from build123d import *

# Parameters (mm, degrees)
F0_W      = 76.2
F0_H      = 101.6
F1_DEPTH  = 25.4
F2_W      = 76.2
F2_H      = 101.6
F2_R      = 6.35
F3_DEPTH  = 25.4
F4_W      = 25.4
F4_H      = 50.8
F6_W      = 18.3004425924
F6_H      = 12.7
F8_R      = 2.54
F9_SIZE   = 2.54
F10_DEPTH = 25.4


with BuildPart() as f1:
    # F0 (on Top) → F1 (new body)
    with BuildSketch(Plane.XY):
        Rectangle(F0_W, F0_H)
    extrude(amount=F1_DEPTH)

    # F2 (on face) → F3 (join)
    with BuildSketch(Plane.XY.offset(25.4)):
        Rectangle(F2_W, F2_H)
        with Locations((-25.4, -38.1)):
            Circle(F2_R, mode=Mode.SUBTRACT)
        with Locations((25.4, -38.1)):
            Circle(F2_R, mode=Mode.SUBTRACT)
        with Locations((-25.4, 38.1)):
            Circle(F2_R, mode=Mode.SUBTRACT)
        with Locations((25.4, 38.1)):
            Circle(F2_R, mode=Mode.SUBTRACT)
        with Locations((-25.4, 38.1)):
            Circle(F2_R)
    extrude(amount=F3_DEPTH)

    # F4 (on Front) → F5 (revolve)
    with BuildSketch(Plane.XZ):
        with Locations((-12.7, 76.2)):
            Rectangle(F4_W, F4_H)
    revolve(axis=Axis((0, 0, 76.2), (0, 0, -1)))

    # F6 (on Front) → F7 (revolve, cut)
    with BuildSketch(Plane.XZ):
        with Locations((-26.9302212962, 76.2)):
            Rectangle(F6_W, F6_H)
    revolve(axis=Axis((0, 0, 101.6), (0, 0, -1)), mode=Mode.SUBTRACT)

    # F8
    f8_edges = [f1.edges().sort_by_distance(p)[0] for p in [
        (25.4, 0, 101.6),
        (25.4, 0, 50.8),
    ]]
    fillet(f8_edges, radius=F8_R)

    # F9
    f9_edges = [f1.edges().sort_by_distance(p)[0] for p in [
        (0, -50.8, 50.8),
        (38.1, 0, 50.8),
        (0, 50.8, 50.8),
        (-38.1, 0, 50.8),
    ]]
    chamfer(f9_edges, length=F9_SIZE)

    # F2 (on face) → F10 (cut)
    with BuildSketch(Plane.XY.offset(25.4)):
        with Locations((-25.4, 38.1)):
            Circle(F2_R)
        with Locations((25.4, 38.1)):
            Circle(F2_R)
        with Locations((-25.4, -38.1)):
            Circle(F2_R)
        with Locations((25.4, -38.1)):
            Circle(F2_R)
    extrude(amount=F10_DEPTH, mode=Mode.SUBTRACT)


solid = f1.part
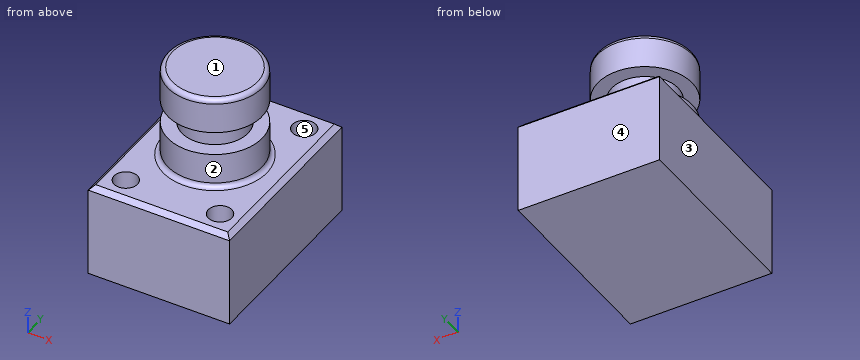
Part model, mm, in its own coordinate system. Face numbers are marked on the shaded views. A direction names the side the tool comes from. Give positions to 0.01 mm unless a question says otherwise; leave off trailing zeros. Loops run counter-clockwise (first coordinate to the right, second up) from the corner with the lowest first, then second, coordinate; pieces in that order, holes last. Notation, with made-up numbers: M -2.75,-18.5 L 25.25,-18.5 A15 ccw 25.25,4.5 Z; hole C 44,56.5 d7. An arc over 180 degrees is marked long. Put each result on its own line as item: value. Start each with the question number.
1) Probe probe 1 along Y at (x, z) = (-25, 33); probe 2 along X at (y, z) = (-38, 40); probe 3 along Z at (x, y) = (18, -1.5). List the from-to ranges inside material, lowest first.
2) Flat gauge pins, fed straight in: pin 1 (14.5 mm diameter, centred on x = -25.4, y = -38.1, fed in from -Z); pin 2 (10 mm diameter, centred on x = 0, z = 65, fed in from -Y); pin 3 (10 mm diameter, centred on x = -28, y = -38, fed in from +Z); pin 4 (6.5 mm diameter, centred on x = 28, y = -36.5, fed in from +Z). Where does each tip first touch, or does it go through?
3) Pull direction X, two halves, no side cores. Call the marked faces 3, 4 and 5: +X half, -X half, draft (parallel to the pull), parting line (faces both ways), or undercut.
4) Saw through at C-C (y = 30). List the corners of the cut face in (x, z).
5) Saw through at D-D (z = 58). List the corners of the cut face in (x, y).
6) Saw through at B-B (z = 79). List the corners of the cut face in (x, y).
7) 3-axis set-ups, long thin cutter, end or side, ignore diameter. For the marked faces 1 and 2: which of +Z, -Z, +X, -X, +Y, -Y reach the whole face in a straight line?
8) Saw through at A-A (y = 0). List the corners of the cut face in (x, z).
Numbers:
1. probe 1: -50.8 to -44.44, -31.76 to 31.76, 44.44 to 50.8
1. probe 2: -38.1 to -31.75, -19.05 to 19.05, 31.75 to 38.1
1. probe 3: 0 to 69.85, 82.55 to 101.6
2. pin 1: z = 0
2. pin 2: y = -25.4
2. pin 3: z = 50.8
2. pin 4: z = 25.4
3. face 3: -X half
3. face 4: draft
3. face 5: undercut
4. outline: M -38.1,0 L 38.1,0 L 38.1,48.26 L 35.56,50.8 L -35.56,50.8 L -38.1,48.26 Z
5. outline: C 0,0 d50.8
6. outline: C 0,0 d35.56
7. face 1: +Z, +X, -X, +Y, -Y
7. face 2: +Z
8. outline: M -38.1,0 L 38.1,0 L 38.1,48.26 L 35.56,50.8 L 27.94,50.8 A2.54 cw 25.4,53.34 L 25.4,69.85 L 17.78,69.85 L 17.78,82.55 L 25.4,82.55 L 25.4,99.06 A2.54 ccw 22.86,101.6 L -22.86,101.6 A2.54 ccw -25.4,99.06 L -25.4,82.55 L -17.78,82.55 L -17.78,69.85 L -25.4,69.85 L -25.4,53.34 A2.54 cw -27.94,50.8 L -35.56,50.8 L -38.1,48.26 Z
